Input: part model. Units: mm. Frame: model coordinates. Face numbers are marked on the shaded views. A direction names the side the tool comes from. Round coordinates to 2 decimals unless told otherwise and drop trailing zeros. Order: outer loops, then holes, each group sorted by start corner. A loop starts at its lowest first (then second) coordinate and runs counter-clockwise, first axis right, second up. Notation, with made-up numbers: (-4.75, -15.75) -> (1.25, -15.75) arc R30 cw to (1.25, 9.25) -> close; hole circle Ø3 at (42, 72.25). An arc over 180 degrees is marked (long way). Use a Markdown table: item, result.
from build123d import *

# Parameters (mm, degrees)
SKETCH1_R             = 6
SKETCH1_R_2           = 3.25
BOSS_EXTRUDE1_DEPTH   = 4
CHAMFER1_SIZE         = 7
CHAMFER2_SIZE         = 13
CHAMFER3_SIZE         = 2
M4_TAPPED_HOLE1_D     = 3.3
M4_TAPPED_HOLE1_DEPTH = 10.1
M4_TAPPED_HOLE1_TIP   = 0.991420021
M3_TAPPED_HOLE1_D     = 2.5
M3_TAPPED_HOLE1_DEPTH = 7.5
M3_TAPPED_HOLE1_TIP   = 0.751075774


with BuildPart() as part:
    # Sketch1 → Boss-Extrude1 (new body)
    with BuildSketch(Plane.XY):
        Polygon((-22.131578947, 33.105263158), (10.368421053, 33.105263158), (10.368421053, -24.394736842), (-7.131578947, -24.394736842), (-7.131578947, -44.394736842), (-22.131578947, -44.394736842), align=None)
        with Locations((-8.631578947, -10.578947368)):
            Circle(SKETCH1_R, mode=Mode.SUBTRACT)
        with Locations((-8.631578947, 26.657894737)):
            Circle(SKETCH1_R_2, mode=Mode.SUBTRACT)
        with BuildLine():
            Line((3.368421053, 11.855263158), (7.368421053, 11.855263158))
            ThreePointArc((7.368421053, 11.855263158), (9.118421053, 10.105263158), (7.368421053, 8.355263158))
            Line((7.368421053, 8.355263158), (3.368421053, 8.355263158))
            ThreePointArc((3.368421053, 8.355263158), (1.618421053, 10.105263158), (3.368421053, 11.855263158))
        make_face(mode=Mode.SUBTRACT)
    extrude(amount=BOSS_EXTRUDE1_DEPTH)

    # Chamfer1
    chamfer1_edges = [part.edges().sort_by_distance(p)[0] for p in [
        (-22.131578947, 33.105263158, 2),
    ]]
    chamfer(chamfer1_edges, length=CHAMFER1_SIZE)

    # Chamfer2
    chamfer2_edges = [part.edges().sort_by_distance(p)[0] for p in [
        (10.368421053, 33.105263158, 2),
        (10.368421053, -24.394736842, 2),
    ]]
    chamfer(chamfer2_edges, length=CHAMFER2_SIZE)

    # Chamfer3
    chamfer3_edges = [part.edges().sort_by_distance(p)[0] for p in [
        (-7.131578947, -44.394736842, 2),
        (-22.131578947, -44.394736842, 2),
    ]]
    chamfer(chamfer3_edges, length=CHAMFER3_SIZE)

    # M4 Tapped Hole1
    with Locations(Plane.XY.offset(4)):
        with Locations((-8.631578947, 15.105263158)):
            Hole(M4_TAPPED_HOLE1_D / 2, depth=M4_TAPPED_HOLE1_DEPTH)
            with Locations((0, 0, -(M4_TAPPED_HOLE1_DEPTH + M4_TAPPED_HOLE1_TIP / 2))):  # 118° drill point
                Cone(0, M4_TAPPED_HOLE1_D / 2, M4_TAPPED_HOLE1_TIP, mode=Mode.SUBTRACT)

    # M3 Tapped Hole1
    with Locations(Plane.XY.offset(4)):
        with Locations((-8.631578947, -1.394736842), (-8.631578947, -20.394736842), (-14.631578947, -29.394736842), (-14.631578947, -39.394736842)):
            Hole(M3_TAPPED_HOLE1_D / 2, depth=M3_TAPPED_HOLE1_DEPTH)
            with Locations((0, 0, -(M3_TAPPED_HOLE1_DEPTH + M3_TAPPED_HOLE1_TIP / 2))):  # 118° drill point
                Cone(0, M3_TAPPED_HOLE1_D / 2, M3_TAPPED_HOLE1_TIP, mode=Mode.SUBTRACT)


solid = part.part
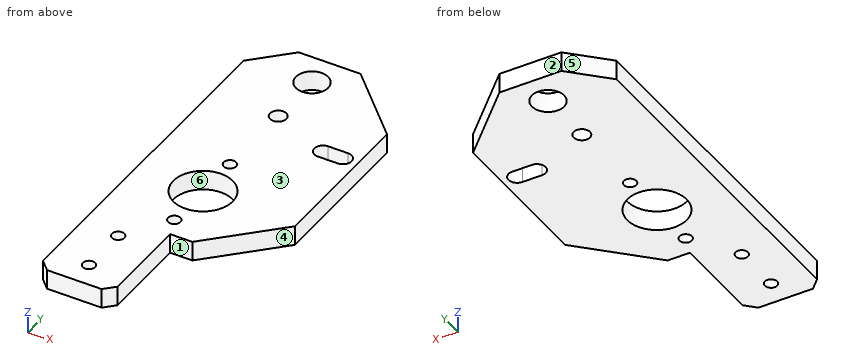
1) Pin query (flat end, axial travel): pin 1 Ø2 at (x, z) = (6, 2) entering from -Y; pin 2 Ø2 at (y, z) = (-31, 2) entering from +X; pin 3 Ø12 at (x, y) = (-1.5, 21.5) entering from -Z. Return the tip coordinate at first contact, or that it passes through.
Results found:
| item | result |
|---|---|
| pin 1 | stops at y = -16.76 |
| pin 2 | stops at x = -7.13 |
| pin 3 | stops at z = 0 |
2) Pull-direction query (Y, two-part tool) for the marked faces 3, 4, 5 and 6; classes: +Y half, -Y half, draft (parallel to the pull), parting line (faces both ways), or undercut.
Results found:
| item | result |
|---|---|
| face 3 | draft |
| face 4 | -Y half |
| face 5 | +Y half |
| face 6 | undercut |
3) Cut plane B-B on z = 2.3. Count the separate pieces of the cut face and the enclosed holes in it, and give its area (3 significant figures).
Results found:
| item | result |
|---|---|
| separate pieces | 1 |
| enclosed holes | 8 |
| area | 1,770 mm² |
4) Cut plane C-C on x = -18. Return loops of the section in (y, z), and give its area (3 significant figures).
Results found:
| item | result |
|---|---|
| outline | (-44.39, 0) -> (30.24, 0) -> (30.24, 4) -> (-44.39, 4) -> close |
| area | 299 mm² |
5) Line query: L1, parallel to Y at x = -10.5, z = 2.05; L2, parallel to X at y = -41, z = 0.3; L3, parallel to X at y = 28.5, z = 1. Output: solid intervals per line, ascending. Write a range as [from, to].
Results found:
| item | result |
|---|---|
| L1 | y = [-44.39, -16.28], [-4.88, 24], [29.32, 33.11] |
| L2 | x = [-22.13, -7.13] |
| L3 | x = [-19.74, -11.31], [-5.95, 1.97] |
6) Set-up query: the marked faces 1 and 2. Return all of +Z, -Z, +X, -X, +Y, -Y with unobstructed straight access to the full face (end or side cutting, diameter ignored); none if empty.
Results found:
| item | result |
|---|---|
| face 1 | +Z, -Z, +X, -Y |
| face 2 | +Z, -Z, +X, -X, +Y |
7) Cut plane A-A on y = -6.5. Return loops of the section in (x, z).
Results found:
| item | result |
|---|---|
| outline | (-22.13, 0) -> (-13.03, 0) -> (-13.03, 4) -> (-22.13, 4) -> close; (-4.23, 0) -> (10.37, 0) -> (10.37, 4) -> (-4.23, 4) -> close |
8) Cut plane D-D on y = 21. Return loops of the section in (x, z), and give its area (3 significant figures).
Results found:
| item | result |
|---|---|
| outline | (-22.13, 0) -> (9.47, 0) -> (9.47, 4) -> (-22.13, 4) -> close |
| area | 126 mm² |
